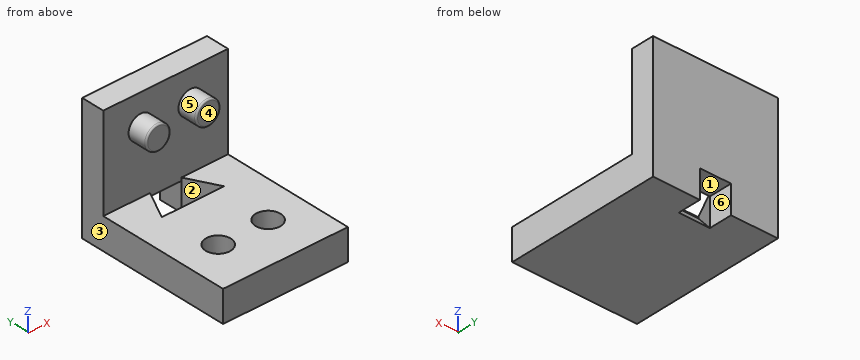
from build123d import *

# Parameters (mm, degrees)
F0_W      = 101.6
F0_H      = 127
F1_DEPTH  = 25.4
F2_R      = 10.16
F3_DEPTH  = 19.05
F4_W      = 19.05
F4_H      = 76.2
F5_DEPTH  = 101.6
F6_R      = 9.906
F7_DEPTH  = 15.875
F8_R      = 1.27
F10_DEPTH = 25.401
F11_W     = 25.4
F11_H     = 22.863189
F12_DEPTH = 25.4
F14_DEPTH = 101.6


with BuildPart() as f1:
    # F0 (on Top) → F1 (new body)
    with BuildSketch(Plane.XY):
        with Locations((50.8, 63.5)):
            Rectangle(F0_W, F0_H)
    extrude(amount=F1_DEPTH)

    # F2 (on face) → F3 (cut)
    with BuildSketch(Plane.XY.offset(25.4)):
        with Locations((30.48, 38.1)):
            Circle(F2_R)
        with Locations((71.12, 38.1)):
            Circle(F2_R)
    extrude(amount=-F3_DEPTH, mode=Mode.SUBTRACT)

    # F4 (on face) → F5 (join)
    with BuildSketch(Plane.YZ.offset(101.6)):
        with Locations((117.475, 63.5)):
            Rectangle(F4_W, F4_H)
    extrude(amount=-F5_DEPTH)

    # F6 (on face) → F7 (join)
    with BuildSketch(Plane.XZ.offset(-107.95)):
        with Locations((30.48, 76.2)):
            Circle(F6_R)
        with Locations((71.12, 76.2)):
            Circle(F6_R)
    extrude(amount=F7_DEPTH)

    # F8
    f8_edges = [f1.edges().sort_by_distance(p)[0] for p in [
        (61.214, 92.075, 76.2),
        (20.574, 92.075, 76.2),
    ]]
    fillet(f8_edges, radius=F8_R)

    # F9 (on face) → F10 (cut, through all)
    with BuildSketch(Plane.XY.offset(25.4)):
        Polygon((63.5, 107.95), (38.1, 107.95), (25.4, 83.384298), (76.2, 83.384298), align=None)
    extrude(amount=-F10_DEPTH, mode=Mode.SUBTRACT)

    # F11 (on face) → F12 (cut)
    with BuildSketch(Plane(origin=(0, 127, 0), x_dir=(-1, 0, 0), z_dir=(0, 1, 0))):
        with Locations((-50.8, 11.431594)):
            Rectangle(F11_W, F11_H)
    extrude(amount=-F12_DEPTH, mode=Mode.SUBTRACT)

    # F13 (on face) → F14 (join)
    with BuildSketch(Plane.YZ.offset(101.6)):
        Polygon((82.55, 0), (107.95, 0), (82.55, 25.4), align=None)
    extrude(amount=-F14_DEPTH)


solid = f1.part
Here's how the part is built. I have some questions about the finished solid (model axes, mm). Face numbers are marked on the shaded views. A direction names the side the tool comes from. Coordinates: 2 decimals unless noted, no trailing zeros. Loops run counter-clockwise (first coordinate to the right, second up) from the corner with the lowest first, then second, coordinate; pieces in that order, holes last. Notation, with made-up numbers: (-28.75, -40) -> (29.25, -40) arc R25 ccw to (29.25, -8) -> close; hole circle Ø2 at (36, 50.5). An arc over 180 degrees is marked (long way). Use one line per item in the form item = value. Start each with the question number.
(1) If we section it at A-A (x = 57.5): Please give me the cut outline in (y, z), then the cut area to 3 significant figures.
(2) On a 3-axis mill with a long thin cutter (end or side, diameter ignored), from which of +Z, -Z, +X, -X, +Y, -Y can I reach the whole of each face in a straight line? I mean the marked faces 4, 5 and 6. Say none if no direction works.
(3) Please list where these lines run through material, in increasing order: line 1 along X through (y, z) = (38, 19); line 2 along Y through (x, z) = (30.48, 16); line 3 along Y through (x, z) = (30, 15).
(4) If we section it at C-C (z = 13): Please give me the cut outline in (x, y).
(5) If we section it at B-B (y = 100.5): Please give me the cut outline in (x, z), then the cut area to 3 significant figures.
(6) Will these pins go through, and if not, where does the flat tip stop? pin 1 (10 mm diameter, centred on x = 70.5, y = 33.5, fed in from +Z); pin 2 (3 mm diameter, centred on x = 19.5, z = 51.5, fed in from -Y); pin 3 (14 mm diameter, centred on x = 72, z = 78, fed in from -Y) (3 decimals).
(7) If we section it at D-D (z = 76.2): Please give me the cut outline in (x, y) (3 decimals).
(8) We'd pull the mould along Z, two halves only. Please class the marked faces 1, 2 and 3: pulls with the +Z half, pulls with the -Z half, needs draft (parallel to the pull), parting line crosses it, or undercut.
Verdict:
q1.outline = (0, 0) -> (107.95, 0) -> (83.38, 24.57) -> (83.38, 25.4) -> (0, 25.4) -> close; (107.95, 22.86) -> (127, 22.86) -> (127, 101.6) -> (107.95, 101.6) -> close
q1.area = 3,920 mm²
q2.face_4 = +Z, +X, -X, -Y
q2.face_5 = -Y
q2.face_6 = -Z, +Y
q3.line_1 = 0 to 20.32, 40.64 to 60.96, 81.28 to 101.6
q3.line_2 = 0 to 27.94, 48.26 to 91.95, 93.21 to 127
q3.line_3 = 0 to 27.95, 48.25 to 127
q4.outline = (0, 0) -> (101.6, 0) -> (101.6, 127) -> (63.5, 127) -> (63.5, 107.95) -> (70.22, 94.95) -> (31.38, 94.95) -> (38.1, 107.95) -> (38.1, 127) -> (0, 127) -> close; hole circle Ø20.32 at (30.48, 38.1); hole circle Ø20.32 at (71.12, 38.1)
q5.outline = (0, 0) -> (101.6, 0) -> (101.6, 25.4) -> (67.35, 25.4) -> (67.35, 7.45) -> (34.25, 7.45) -> (34.25, 25.4) -> (0, 25.4) -> close; circle Ø19.81 at (30.48, 76.2); circle Ø19.81 at (71.12, 76.2)
q5.area = 2,600 mm²
q6.pin_1 = 6.35
q6.pin_2 = 107.95
q6.pin_3 = 92.075
q7.outline = (0, 107.95) -> (20.574, 107.95) -> (20.574, 93.345) arc R1.27 ccw to (21.844, 92.075) -> (39.116, 92.075) arc R1.27 ccw to (40.386, 93.345) -> (40.386, 107.95) -> (61.214, 107.95) -> (61.214, 93.345) arc R1.27 ccw to (62.484, 92.075) -> (79.756, 92.075) arc R1.27 ccw to (81.026, 93.345) -> (81.026, 107.95) -> (101.6, 107.95) -> (101.6, 127) -> (0, 127) -> close
q8.face_1 = pulls with the -Z half
q8.face_2 = undercut
q8.face_3 = needs draft
